The listing builds one solid part. Answer for the finished solid, in the listing's coordinates (mm). Face numbers are marked on the shaded views. Coordinates: 2 decimals unless noted, no trailing zeros. Order: outer loops, then holes, each group sorted by start corner. A loop starts at its lowest first (then second) coordinate and runs counter-clockwise, first axis right, second up. Notation, with made-up numbers: (6.5, -15.75) -> (46.5, -15.75) arc R24 cw to (46.5, 11.25) -> close; hole circle Ø1 at (19, 61). An arc over 180 degrees is marked (long way). Answer in a Markdown table with one row per item.
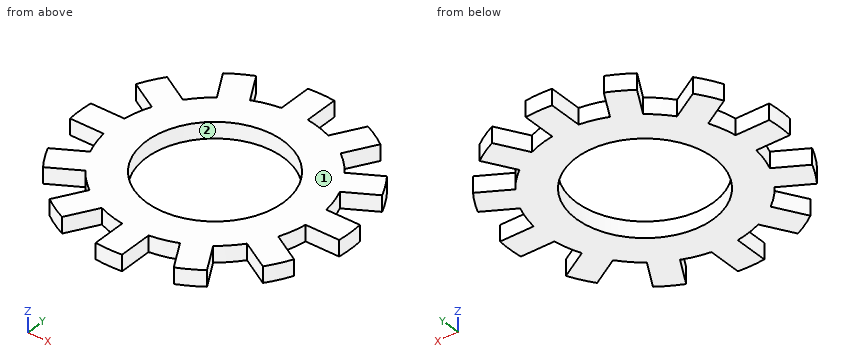
```python
from build123d import *

# Parameters (mm, degrees)
SKETCH1_R         = 3.2
SKETCH1_R_2       = 2.15
EXTRUDE1_DEPTH    = 0.5
EXTRUDE2_DEPTH    = 0.5
CIRPATTERN1_COUNT = 12


with BuildPart() as part:
    # Sketch1 → Extrude1 (new body)
    with BuildSketch(Plane.XY):
        Circle(SKETCH1_R)
        Circle(SKETCH1_R_2, mode=Mode.SUBTRACT)
    extrude(amount=EXTRUDE1_DEPTH)

    # Sketch2 → Extrude2 (add)
    with BuildSketch(Plane.XY):
        with BuildLine():
            Line((-0.414110472, 4.229776887), (-0.414110472, 3.173091949))
            Line((-0.414110472, 3.173091949), (0.414110472, 3.173091949))
            Line((0.414110472, 3.173091949), (0.414110472, 4.229776887))
            ThreePointArc((0.414110472, 4.229776887), (0, 4.25), (-0.414110472, 4.229776887))
        make_face()
    extrude2 = extrude(amount=EXTRUDE2_DEPTH)

    # CirPattern1: Extrude2 ×12 about axis
    cirpattern1_axis = Axis((0, 0, 0), (0, 0, 1))
    for i in range(1, CIRPATTERN1_COUNT):
        add(extrude2.rotate(cirpattern1_axis, i * 360 / CIRPATTERN1_COUNT))


solid = part.part
```
(1) A cutting plane is placed at A-A, the plane x = 0. Determine the outline of the cut face in (y, z), then the cut area to 3 significant figures.
Check values:
| item | result |
|---|---|
| outline | (-4.25, 0) -> (-2.15, 0) -> (-2.15, 0.5) -> (-4.25, 0.5) -> close; (2.15, 0) -> (4.25, 0) -> (4.25, 0.5) -> (2.15, 0.5) -> close |
| area | 2.10 mm² |
(2) For a pull along X with two mould halves and no side action, classify the marked faces 1 and 2 as released by +X, released by -X, zero draft, split by the parting line, or undercut.
Check values:
| item | result |
|---|---|
| face 1 | zero draft |
| face 2 | undercut |
(3) A flat-ended cylindrical pin translates along its axis: pin 1 (1 mm diameter, centred on x = -0.5, y = -1.5, fed in from +Z). Find the tip coordinate at first contact, or state that the pin passes through.
Check values:
| item | result |
|---|---|
| pin 1 | through |
(4) A cutting plane is placed at C-C, the plane x = -2.75. Determine the outline of the cut face in (y, z), then the cut area to 3 significant figures.
Check values:
| item | result |
|---|---|
| outline | (-2.07, 0) -> (2.07, 0) -> (2.07, 0.5) -> (-2.07, 0.5) -> close |
| area | 2.07 mm² |
(5) Find the intervals of material crossed by line 1 along Y through (x, z) = (0, 0.15); line 2 along Y through (x, z) = (-3.5, 0.45); line 3 along X through (y, z) = (2.25, 0.25), in increasing order. Write a range as from..to.
Check values:
| item | result |
|---|---|
| line 1 | -4.25..-2.15, 2.15..4.25 |
| line 2 | -2.41..-1.54, -0.41..0.41, 1.54..2.41 |
| line 3 | -3.61..-3.07, -2.28..2.28, 3.07..3.61 |
